```python
from build123d import *

# Parameters (mm, degrees)
F0_R      = 70
F1_DEPTH  = 180
F2_R      = 65
F3_DEPTH  = 40
F5_R      = 15
F5_R_2    = 12.5
F5_R_3    = 10
F6_DEPTH  = 125
F8_R      = 65
F9_DEPTH  = 130
F10_R     = 2.5
F11_DEPTH = 2


with BuildPart() as f1:
    # F0 (on Top) → F1 (new body)
    with BuildSketch(Plane.XY):
        Circle(F0_R)
    extrude(amount=F1_DEPTH)

    # F2 (on face) → F3 (cut)
    with BuildSketch(Plane(origin=(0, 0, 0), x_dir=(1, 0, 0), z_dir=(0, 0, -1))):
        Circle(F2_R)
    extrude(amount=-F3_DEPTH, mode=Mode.SUBTRACT)

    # F5 (on offset) → F6 (cut)
    with BuildSketch(Plane.XY.offset(40)):
        with Locations((40, 0)):
            Circle(F5_R)
        with Locations((-40, 0)):
            Circle(F5_R)
        with Locations((0, 40)):
            Circle(F5_R_2)
        with Locations((0, -40)):
            Circle(F5_R_2)
        with Locations((-28, 28.565714)):
            Circle(F5_R_3)
        with Locations((27.423085, -29.12)):
            Circle(F5_R_3)
        with Locations((-29.12, -27.423085)):
            Circle(F5_R_3)
        with Locations((28.565714, 28)):
            Circle(F5_R_3)
    extrude(amount=F6_DEPTH, mode=Mode.SUBTRACT)

    # F8 (on offset) → F9 (cut)
    with BuildSketch(Plane.XY.offset(45)):
        Circle(F8_R)
    extrude(amount=F9_DEPTH, mode=Mode.SUBTRACT)

    # F10 (on face) → F11 (join)
    with BuildSketch(Plane(origin=(0, 0, 40), x_dir=(1, 0, 0), z_dir=(0, 0, -1))):
        Circle(F10_R)
    extrude(amount=F11_DEPTH)


solid = f1.part
```
The model under review builds one solid part; all positions refer to its coordinate system, in mm. A direction names the side the tool comes from. Round coordinates to 2 decimals unless told otherwise and drop trailing zeros. Loops run counter-clockwise (first coordinate to the right, second up) from the corner with the lowest first, then second, coordinate; pieces in that order, holes last. Notation, with made-up numbers: M -33,-30 L -17,-30 A13 cw -17,-17 Z; hole C -24,-36.5 d2. An arc over 180 degrees is marked long. Write item = value, one per line.
Item 1: Take a section at D-D on x = -29.12. Write out the cut boundary in (y, z).
Return value:
outline = M -63.66,0 L -58.11,0 L -58.11,40 L -37.42,40 L -37.42,45 L -58.11,45 L -58.11,175 L 58.11,175 L 58.11,45 L 38.5,45 L 38.5,40 L 58.11,40 L 58.11,0 L 63.66,0 L 63.66,180 L -63.66,180 Z; M -17.42,40 L -10.33,40 L -10.33,45 L -17.42,45 Z; M 10.33,40 L 18.63,40 L 18.63,45 L 10.33,45 Z
Item 2: The part is to be moulded in two halves that separate along X. For faces 4 (the cylindrical face through (-29.3, 38.48, 42.46)), 5 (the flat face through (-1, 1, 180)), 6 (the cylindrical face through (-55.55, -42.594, 88.74)), say which applies: released by +X, released by -X, zero draft, split by the parting line, or undercut.
Return value:
face_4 = undercut
face_5 = zero draft
face_6 = split by the parting line
Item 3: Insertion check: P1, Ø10, axis at y = -34, z = 156, coming from the +X side; P2, Ø5, axis at y = -16.5, z = 66.5, coming from the +X side; P3, Ø6, axis at x = 16, y = -55, coming from the -Z side. Each pin has a flat end and moves straight along its axis. Give the tip position at first contact, or say it passes through.
Return value:
P1 = 63.71
P2 = 68.59
P3 = 40
Item 4: For line 1 (Y direction, x = 0, z = 41); line 2 (Z direction, x = -23, y = -59); line 3 (Y direction, x = 0, z = 95), list the stretches that pass through material, from the lowest coordinate up. Write a range as [from, to].
Return value:
line_1 = [-70, -52.5], [-27.5, 27.5], [52.5, 70]
line_2 = [40, 45], [175, 180]
line_3 = [-70, -65], [65, 70]
Item 5: Take a section at B-B on y = -9. Write out the cut boundary in (x, z), then the cut area to 3 significant figures.
Return value:
outline = M -69.42,0 L -64.37,0 L -64.37,40 L -52,40 L -52,45 L -64.37,45 L -64.37,175 L 64.37,175 L 64.37,45 L 52,45 L 52,40 L 64.37,40 L 64.37,0 L 69.42,0 L 69.42,180 L -69.42,180 Z; M -28,40 L 28,40 L 28,45 L -28,45 Z
area = 2,860 mm2
Item 6: Take a section at C-C on y = 34.5. Write out the cut boundary in (x, z), then the cut area to 3 significant figures.
Return value:
outline = M -60.91,0 L -55.09,0 L -55.09,40 L -36.05,40 L -36.05,45 L -55.09,45 L -55.09,175 L 55.09,175 L 55.09,45 L 36.17,45 L 36.17,40 L 55.09,40 L 55.09,0 L 60.91,0 L 60.91,180 L -60.91,180 Z; M -19.95,40 L -11.22,40 L -11.22,45 L -19.95,45 Z; M 11.22,40 L 20.97,40 L 20.97,45 L 11.22,45 Z
area = 2,930 mm2
Item 7: Machinability: for faces 1 (the flat face through (-1, 1, 45)), 2 (the flat face through (20.4, -61.9, 0)), 3 (the cylindrical face through (-39.11, -26.98, 42.46)), which of the approach directions +Z, -Z, +X, -X, +Y, -Y give a long, thin tool a straight path to every point of the face, cutting with its end or side? Answer none if there is none.
Return value:
face_1 = none
face_2 = -Z, +X, -X, +Y, -Y
face_3 = -Z
Item 8: Take a section at A-A on x = 0. Write out the cut boundary in (y, z).
Return value:
outline = M -70,0 L -65,0 L -65,40 L -52.5,40 L -52.5,45 L -65,45 L -65,175 L 65,175 L 65,45 L 52.5,45 L 52.5,40 L 65,40 L 65,0 L 70,0 L 70,180 L -70,180 Z; M -27.5,40 L -2.5,40 L -2.5,38 L 2.5,38 L 2.5,40 L 27.5,40 L 27.5,45 L -27.5,45 Z
